For this review, take the finished solid that the model builds, in its own axes (mm). Face numbers are marked on the shaded views. Coordinates: 2 decimals unless noted, no trailing zeros. Loops run counter-clockwise (first coordinate to the right, second up) from the corner with the lowest first, then second, coordinate; pieces in that order, holes last. Notation, with made-up numbers: (68.5, 87.25) -> (114.5, 87.25) arc R15 ccw to (114.5, 91.25) -> close; hole circle Ø4 at (15.5, -33.75). An arc over 180 degrees is marked (long way). Answer in a Markdown table with one row per item.
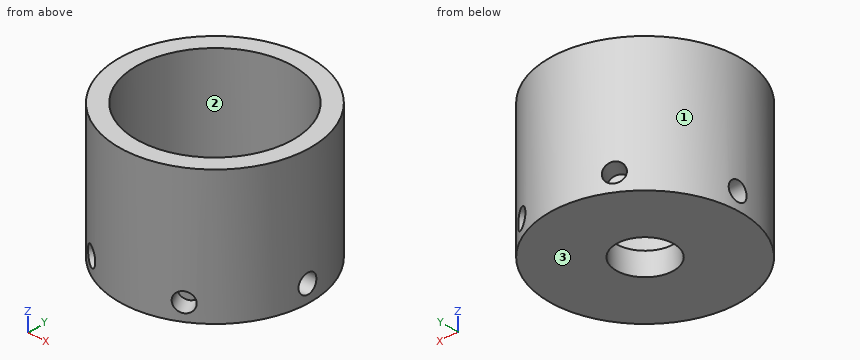
from build123d import *

# Parameters (mm, degrees)
F0_R             = 25
F1_DEPTH         = 35
F2_R             = 20.5
F3_DEPTH         = 27
F4_R             = 7.5
F5_DEPTH         = 8.001
F6_R             = 13.5
F7_DEPTH         = 2
F10_R            = 2.5
F11_DEPTH        = 5
F11_COPIES_COUNT = 6


# Not quite as in the source:
# - a pattern or mirror of a feature is missing from the dataset's text; its kind, count and spacing are read off the source's solid


with BuildPart() as f1:
    # F0 (on Top) → F1 (new body)
    with BuildSketch(Plane.XY):
        with Locations((0, 6.5720938146)):
            Circle(F0_R)
    extrude(amount=F1_DEPTH)

    # F2 (on face) → F3 (cut)
    with BuildSketch(Plane.XY.offset(35)):
        with Locations((0, 6.5720938146)):
            Circle(F2_R)
    extrude(amount=-F3_DEPTH, mode=Mode.SUBTRACT)

    # F4 (on face) → F5 (cut, through all)
    with BuildSketch(Plane.XY.offset(8)):
        with Locations((0, 6.5720938146)):
            Circle(F4_R)
    extrude(amount=-F5_DEPTH, mode=Mode.SUBTRACT)

    # F6 (on face) → F7 (cut)
    with BuildSketch(Plane.XY.offset(8)):
        with Locations((0, 6.5720938146)):
            Circle(F6_R)
    extrude(amount=-F7_DEPTH, mode=Mode.SUBTRACT)

    # F10 (on offset) → F11 (cut)
    with BuildSketch(Plane.YZ.offset(25)):
        with Locations((6.071, 4.5)):
            Circle(F10_R)
    f11 = extrude(amount=-F11_DEPTH, mode=Mode.SUBTRACT)

    # F11_copies: F11 ×6 about axis
    f11_copies_axis = Axis((0, 6.572094, 0), (0, 0, 1))
    for i in range(1, F11_COPIES_COUNT):
        add(f11.rotate(f11_copies_axis, i * 360 / F11_COPIES_COUNT), mode=Mode.SUBTRACT)


solid = f1.part
Item 1: Insertion check: pin 1 (12.5 mm diameter, centred on x = 3, y = 13, fed in from +Z); pin 2 (10 mm diameter, centred on x = 11, z = 16, fed in from +Y); pin 3 (3 mm diameter, centred on y = 10.5, z = 22.5, fed in from +X). Each pin has a flat end and moves straight along its axis. Give the tip position at first contact, or say it passes through.
Worked answers:
| item | result |
|---|---|
| pin 1 | z = 6 |
| pin 2 | y = 30.84 |
| pin 3 | x = 24.88 |
Item 2: For L1, parallel to X at y = -10.5, z = 3.5; L2, parallel to X at y = 7, z = 4; L3, parallel to X at y = 25, z = 6, list the stretches that pass through material, from the lowest coordinate up.
Worked answers:
| item | result |
|---|---|
| L1 | -18.26 to -13.08, -10.43 to 10.43, 11.92 to 18.26 |
| L2 | -20 to -7.49, 7.49 to 20 |
| L3 | -16.89 to -12.37, -8.08 to 8.91, 13.53 to 16.89 |
Item 3: Take a section at A-A, the plane x = 0. State the section outline as (y, z) points.
Worked answers:
| item | result |
|---|---|
| outline | (-18.43, 0) -> (-0.93, 0) -> (-0.93, 6) -> (-6.93, 6) -> (-6.93, 8) -> (-13.93, 8) -> (-13.93, 35) -> (-18.43, 35) -> close; (14.07, 0) -> (31.57, 0) -> (31.57, 35) -> (27.07, 35) -> (27.07, 8) -> (20.07, 8) -> (20.07, 6) -> (14.07, 6) -> close |
Item 4: The part is to be moulded in two halves that separate along X. For the marked faces 1, 2 and 3, say which applies: +X half, -X half, draft (parallel to the pull), parting line (faces both ways), or undercut.
Worked answers:
| item | result |
|---|---|
| face 1 | parting line |
| face 2 | undercut |
| face 3 | draft |
Item 5: Take a section at D-D, the plane y = 16. State the section outline as (x, z) points, and give its area (3 significant figures).
Worked answers:
| item | result |
|---|---|
| outline | (-23.15, 0) -> (23.15, 0) -> (23.15, 35) -> (18.2, 35) -> (18.2, 8) -> (9.66, 8) -> (9.66, 6) -> (-9.66, 6) -> (-9.66, 8) -> (-18.2, 8) -> (-18.2, 35) -> (-23.15, 35) -> close |
| area | 599 mm² |
Item 6: Take a section at C-C, the plane y = 10.5. State the section outline as (x, z) points, and give its area (3 significant figures).
Worked answers:
| item | result |
|---|---|
| outline | (-24.69, 0) -> (-6.39, 0) -> (-6.39, 6) -> (-12.92, 6) -> (-12.92, 8) -> (-20.12, 8) -> (-20.12, 35) -> (-24.69, 35) -> close; (6.39, 0) -> (24.69, 0) -> (24.69, 35) -> (20.12, 35) -> (20.12, 8) -> (12.92, 8) -> (12.92, 6) -> (6.39, 6) -> close |
| area | 513 mm² |
Item 7: Take a section at B-B, the plane z = 4.5. State the section outline as (x, y) points, and give its area (3 significant figures).
Worked answers:
| item | result |
|---|---|
| outline | (-24.92, 4.57) arc R25 ccw to (-15.01, -13.42) -> (-12.6, -9.25) -> (-8.27, -11.75) -> (-10.73, -16.01) arc R25 ccw to (9.81, -16.42) -> (7.4, -12.25) -> (11.73, -9.75) -> (14.19, -14.01) arc R25 ccw to (24.82, 3.57) -> (20, 3.57) -> (20, 8.57) -> (24.92, 8.57) arc R25 ccw to (15.01, 26.57) -> (12.6, 22.39) -> (8.27, 24.89) -> (10.73, 29.15) arc R25 ccw to (-9.81, 29.57) -> (-7.4, 25.39) -> (-11.73, 22.89) -> (-14.19, 27.15) arc R25 ccw to (-24.82, 9.57) -> (-20, 9.57) -> (-20, 4.57) -> close; hole circle Ø15 at (0, 6.57) |
| area | 1,640 mm² |
